from build123d import *

# Parameters (mm, degrees)
SKETCH1_R           = 21.5
BOSS_EXTRUDE1_DEPTH = 22
SKETCH3_R           = 15
CUT_EXTRUDE1_DEPTH  = 22
SKETCH4_R           = 17
CUT_EXTRUDE2_DEPTH  = 2
CUT_EXTRUDE3_START  = -2
SKETCH5_R           = 17
CUT_EXTRUDE3_DEPTH  = 2
CHAMFER1_SIZE       = 0.5
CHAMFER3_SIZE       = 0.5
CHAMFER3_SIZE2      = 1.37373871
CHAMFER5_SIZE       = 0.5
CHAMFER5_SIZE2      = 1.37373871


with BuildPart() as part:
    # Sketch1 → Boss-Extrude1 (new body)
    with BuildSketch(Plane.XY):
        Circle(SKETCH1_R)
    extrude(amount=BOSS_EXTRUDE1_DEPTH)

    # Sketch3 → Cut-Extrude1 (cut)
    with BuildSketch(Plane.XY.offset(22)):
        Circle(SKETCH3_R)
    extrude(amount=-CUT_EXTRUDE1_DEPTH, mode=Mode.SUBTRACT)

    # Sketch4 → Cut-Extrude2 (cut)
    with BuildSketch(Plane.XY.offset(22)):
        Circle(SKETCH4_R)
    extrude(amount=-CUT_EXTRUDE2_DEPTH, mode=Mode.SUBTRACT)

    # Sketch5 → Cut-Extrude3 (cut)
    with BuildSketch(Plane(origin=(0, 0, 0), x_dir=(-1, 0, 0), z_dir=(0, 0, -1)).offset(CUT_EXTRUDE3_START)):
        with Locations(Location((0, 0, 0), (0, 0, 180))):
            Circle(SKETCH5_R)
    extrude(amount=CUT_EXTRUDE3_DEPTH, mode=Mode.SUBTRACT)

    # Chamfer1
    chamfer1_edges = [part.edges().sort_by_distance(p)[0] for p in [
        (-17, 0, 22),
        (-17, 0, 0),
    ]]
    chamfer(chamfer1_edges, length=CHAMFER1_SIZE)

    # Chamfer3
    chamfer3_edges = [part.edges().sort_by_distance(p)[0] for p in [
        (-21.5, 0, 0),
    ]]
    chamfer3_side = [part.faces().sort_by_distance(p)[0] for p in [
        (-18.108111832, 0, 0),
    ]]
    chamfer(chamfer3_edges, length=CHAMFER3_SIZE, length2=CHAMFER3_SIZE2, reference=chamfer3_side[0])

    # Chamfer5
    chamfer5_edges = [part.edges().sort_by_distance(p)[0] for p in [
        (-21.5, 0, 22),
    ]]
    chamfer5_side = [part.faces().sort_by_distance(p)[0] for p in [
        (-21.5, 0, 11.686869355),
    ]]
    chamfer(chamfer5_edges, length=CHAMFER5_SIZE, length2=CHAMFER5_SIZE2, reference=chamfer5_side[0])


solid = part.part
Check sheet for the modelled part. Datum: model origin and axes. Units: mm. A direction names the side the tool comes from. Round coordinates to 2 decimals unless told otherwise and drop trailing zeros. Loops run counter-clockwise (first coordinate to the right, second up) from the corner with the lowest first, then second, coordinate; pieces in that order, holes last. Notation, with made-up numbers: M 17,-22 L 35,-22 A18 ccw 35,-7 Z; hole C -1.5,76.25 d2. An arc over 180 degrees is marked long. One line per question, with ' | ' between items. Start each with the question number.
Item 1: Scan lines: probe 1 along Y at (x, z) = (0.5, 14.75); probe 2 along Y at (x, z) = (0, 20.4); probe 3 along X at (y, z) = (6, 18). Record each from-to range of solid material in increasing order.
Item 2: Set-up check for faces 4 (the face through (-2.213, -16.855, 1.26)), 5 (the face through (9.139, 14.334, 20.76)), 6 (the face through (-8, 16, 0)): record each of +Z, -Z, +X, -X, +Y, -Y from which the full face is reachable in a straight line by a thin tool's end or side.
Item 3: Release check for a two-part mould opening along Y. For faces 1 (the face through (6, 14, 2)), 2 (the face through (0, 18, 22)), 3 (the face through (-2.799, 21.317, 11.296)) record: released by +Y, released by -Y, zero draft, split by the parting line, or undercut.
Item 4: Gauge pin test, flat ends, axial feed: pin 1 Ø3 at (y, z) = (10, 16) entering from +X; pin 2 Ø1 at (x, z) = (9.5, 8.5) entering from -Y; pin 3 Ø2 at (y, z) = (2.5, 10.5) entering from +X. Record the tip position at first contact, or that the pin passes through.
Item 5: Section check C-C (z = 14.75). Record the boundary of the cut face in (x, y), and give its area (3 significant figures).
Item 6: Section check A-A (y = 0). Record the boundary of the cut face in (x, z).
Worked out:
1) probe 1: -21.49 to -14.99, 14.99 to 21.49 | probe 2: -21.5 to -17, 17 to 21.5 | probe 3: -20.65 to -13.75, 13.75 to 20.65
2) face 4: -Z | face 5: +Z | face 6: -Z, +X, -X, +Y, -Y
3) face 1: undercut | face 2: zero draft | face 3: split by the parting line
4) pin 1: x = 19.75 | pin 2: y = -19.53 | pin 3: x = 21.45
5) outline: C 0,0 d43; hole C 0,0 d30 | area: 745 mm^2
6) outline: M -21.5,1.37 L -21,0 L -17.5,0 L -17,0.5 L -17,2 L -15,2 L -15,20 L -17,20 L -17,21.5 L -17.5,22 L -20.13,22 L -21.5,21.5 Z; M 15,2 L 17,2 L 17,0.5 L 17.5,0 L 21,0 L 21.5,1.37 L 21.5,21.5 L 20.13,22 L 17.5,22 L 17,21.5 L 17,20 L 15,20 Z
